from build123d import *

# Parameters (mm, degrees)
F0_R      = 3.175
F1_DEPTH  = 1.5875
F6_W      = 20.4342100769
F6_H      = 36.2635273486
F7_DEPTH  = 10.668
F8_R      = 0.25
F9_DEPTH  = 25.4
F10_DEPTH = 26.9875


# Not quite as in the source:
# - a length typed as a fraction of an inch, garbled in the dataset ("3 / 203.2 mm" for 3/8 in), is restored


with BuildPart() as f1:
    # F0 (on Top) → F1 (new body)
    with BuildSketch(Plane.XY):
        Circle(F0_R)
    extrude(amount=F1_DEPTH)

    # F2 (on Front) → F4 (revolve)
    with BuildSketch(Plane.XZ):
        with BuildLine():
            Line((-2.3876, 0), (0, 0))
            Line((0, 0), (0, 9.525))
            ThreePointArc((0, 9.525), (-1.6882881508, 8.8256881508), (-2.3876, 7.1374))
            Line((-2.3876, 7.1374), (-2.3876, 0))
        make_face()
    revolve(axis=Axis((0, 0, 21.5854328126), (0, 0, 1)))

    # F6 (on offset) → F7 (cut)
    with BuildSketch(Plane.XZ.offset(2.7178)):
        with Locations((0.1439033076, 14.3902888522)):
            Rectangle(F6_W, F6_H)
    extrude(amount=F7_DEPTH, mode=Mode.SUBTRACT)

    # F8 (on face) → F9 (join)
    with BuildSketch(Plane(origin=(0, 0, 0), x_dir=(1, 0, 0), z_dir=(0, 0, -1))):
        with Locations((0, -1.4801331563)):
            Circle(F8_R)
        with Locations((0, 1.4801331563)):
            Circle(F8_R)
    extrude(amount=F9_DEPTH)

    # F8 (on face) → F10 (join)
    with BuildSketch(Plane(origin=(0, 0, 0), x_dir=(1, 0, 0), z_dir=(0, 0, -1))):
        with Locations((0, 1.4801331563)):
            Circle(F8_R)
    extrude(amount=F10_DEPTH)


solid = f1.part
Source: CAD feature listing. Evaluate the final solid. Frame: model axes, mm. A direction names the side the tool comes from. Round coordinates to 2 decimals unless told otherwise and drop trailing zeros. Loops run counter-clockwise (first coordinate to the right, second up) from the corner with the lowest first, then second, coordinate; pieces in that order, holes last. Notation, with made-up numbers: M 20.25,-12.5 L 42.25,-12.5 A7 ccw 42.25,-2.5 Z; hole C 8.25,46 d3. An arc over 180 degrees is marked long. Return JSON: item names as keys, results as strings. Group by question number.
1. Material intervals for line 1 along X through (y, z) = (-0.1, 5); line 2 along Z through (x, y) = (1.25, 2.85); line 3 along Z through (x, y) = (1, -0.7), sorted ascending. Write a range as from..to.
2. Pin query (flat end, axial travel): pin 1 (3 mm diameter, centred on y = 2.5, z = -7.5, fed in from +X); pin 2 (1.5 mm diameter, centred on x = -0.5, z = -8.5, fed in from +Y); pin 3 (1.8 mm diameter, centred on x = 1, y = -0.5, fed in from -Z). Return the tip coordinate at first contact, or that it passes through.
3. Section query D-D on z = 0.5. Output: boundary loops of the cut face in (x, y) (3 decimals), and give its area (3 significant figures).
4. Reachability of faces 1 (the face through (-2, 2, 1.588)), 2 (the face through (0.115, 3.173, 0.783)) from +Z, -Z, +X, -X, +Y, -Y: full face, straight path, thin tool, end or side. Return the list, or none.
5. Section query B-B on z = -12.5. Output: boundary loops of the cut face in (x, y), and give its area (3 significant figures).
6. Section query C-C on x = 1.25. Output: boundary loops of the cut face in (y, z).
7. Section query A-A on y = 0. Output: boundary loops of the cut face in (x, z) (1 decimal), and give its area (3 significant figures).
Checks:
{
 "1": {"line 1": "x = -2.39..2.39", "line 2": "z = 0..1.59", "line 3": "z = 0..9.19"},
 "2": {"pin 1": "stops at x = 0.25", "pin 2": "stops at y = 1.73", "pin 3": "stops at z = 0"},
 "3": {"outline": "M -1.641,-2.718 L 1.641,-2.718 A3.175 ccw long Z", "area": "30.7 mm²"},
 "4": {"face 1": "+Z", "face 2": "+Z, -Z"},
 "5": {"outline": "C 0,-1.48 d0.5; C 0,1.48 d0.5", "area": "0.393 mm²"},
 "6": {"outline": "M -2.72,0 L 2.92,0 L 2.92,1.59 L 2.03,1.59 L 2.03,7.14 A2.03 ccw -2.03,7.14 L -2.03,1.59 L -2.72,1.59 Z"},
 "7": {"outline": "M -3.2,0 L 3.2,0 L 3.2,1.6 L 2.4,1.6 L 2.4,7.1 A2.4 ccw -2.4,7.1 L -2.4,1.6 L -3.2,1.6 Z", "area": "45.5 mm²"}
}
